Geometry: final body of the model. Coordinates: model frame, mm. Round coordinates to 2 decimals unless told otherwise and drop trailing zeros. Loops run counter-clockwise (first coordinate to the right, second up) from the corner with the lowest first, then second, coordinate; pieces in that order, holes last. Notation, with made-up numbers: (-4.5, 84) - (51.5, 84) arc R33 cw to (51.5, 112) - close; hole circle Ø6 at (20, 87.25). An arc over 180 degrees is marked (long way). Answer as CSV lines item,"result".
from build123d import *

# Parameters (mm, degrees)
BOSS_EXTRUDE1_DEPTH = 2.54


with BuildPart() as part:
    # Model → Boss-Extrude1 (new body)
    with BuildSketch(Plane.XY):
        with BuildLine():
            Line((0.837402515, 4.194701871), (0.812002515, 4.238232391))
            ThreePointArc((0.812002515, 4.238232391), (0.774103936, 4.334279035), (0.761202515, 4.436723231))
            ThreePointArc((0.761202515, 4.436723231), (0.774103936, 4.539167428), (0.812002515, 4.635214071))
            Line((0.812002515, 4.635214071), (0.837402515, 4.678744591))
            Line((0.837402515, 4.678744591), (0.862802515, 4.715127551))
            Line((0.862802515, 4.715127551), (0.888202515, 4.746935971))
            Line((0.888202515, 4.746935971), (0.913602515, 4.775495731))
            Line((0.913602515, 4.775495731), (0.939002515, 4.801589151))
            Line((0.939002515, 4.801589151), (0.964402515, 4.825726771))
            Line((0.964402515, 4.825726771), (0.989802515, 4.848266731))
            Line((0.989802515, 4.848266731), (1.015202515, 4.869465571))
            ThreePointArc((1.015202515, 4.869465571), (1.089772897, 4.925535764), (1.167602515, 4.976986311))
            Line((1.167602515, 4.976986311), (1.193002515, 4.992508251))
            ThreePointArc((1.193002515, 4.992508251), (1.305754767, 5.055617229), (1.421602515, 5.112845831))
            Line((1.421602515, 5.112845831), (1.447002515, 5.124547611))
            ThreePointArc((1.447002515, 5.124547611), (1.598149319, 5.189132356), (1.751802515, 5.247503931))
            Line((1.751802515, 5.247503931), (1.777202515, 5.256564111))
            ThreePointArc((1.777202515, 5.256564111), (1.991913899, 5.32756087), (2.209002515, 5.390917411))
            Line((2.209002515, 5.390917411), (2.234402515, 5.397856691))
            ThreePointArc((2.234402515, 5.397856691), (2.512823075, 5.468426298), (2.793202515, 5.530759651))
            Line((2.793202515, 5.530759651), (2.818602515, 5.536032691))
            ThreePointArc((2.818602515, 5.536032691), (3.18604982, 5.606262809), (3.555202515, 5.666893491))
            Line((3.555202515, 5.666893491), (3.580602515, 5.670744131))
            ThreePointArc((3.580602515, 5.670744131), (4.049820252, 5.735370933), (4.520402515, 5.789169091))
            Line((4.520402515, 5.789169091), (4.545802515, 5.791795451))
            ThreePointArc((4.545802515, 5.791795451), (5.129518216, 5.845119064), (5.714202515, 5.886491731))
            Line((5.714202515, 5.886491731), (5.739602515, 5.888043671))
            ThreePointArc((5.739602515, 5.888043671), (6.437840457, 5.923508303), (7.136602515, 5.946433191))
            Line((7.136602515, 5.946433191), (7.162002515, 5.947052951))
            ThreePointArc((7.162002515, 5.947052951), (7.987453434, 5.959786425), (8.813002515, 5.959509111))
            Line((8.813002515, 5.959509111), (8.838402515, 5.959313531))
            ThreePointArc((8.838402515, 5.959313531), (9.791045496, 5.944671622), (10.743402515, 5.917119051))
            Line((10.743402515, 5.917119051), (10.768802515, 5.916224971))
            ThreePointArc((10.768802515, 5.916224971), (11.874009843, 5.869976991), (12.978602515, 5.810840371))
            Line((12.978602515, 5.810840371), (13.004002515, 5.809341771))
            ThreePointArc((13.004002515, 5.809341771), (14.249024434, 5.729100435), (15.493202515, 5.636692891))
            Line((15.493202515, 5.636692891), (15.518602515, 5.634691371))
            ThreePointArc((15.518602515, 5.634691371), (16.763614783, 5.531321058), (18.007802486, 5.418458634))
            Line((18.007802486, 5.418458634), (18.134802481, 5.406436814))
            ThreePointArc((18.134802481, 5.406436814), (19.379819615, 5.283861478), (20.624002515, 5.153089591))
            Line((20.624002515, 5.153089591), (20.649402515, 5.150333691))
            ThreePointArc((20.649402515, 5.150333691), (21.894471689, 5.011181274), (23.138602515, 4.863875031))
            Line((23.138602515, 4.863875031), (23.164002515, 4.860781311))
            ThreePointArc((23.164002515, 4.860781311), (24.409193854, 4.704533833), (25.653202485, 4.539133495))
            Line((25.653202485, 4.539133495), (26.161202515, 4.468727231))
            ThreePointArc((26.161202515, 4.468727231), (26.191266445, 4.466787161), (26.189326375, 4.436723231))
            ThreePointArc((26.189326375, 4.436723231), (26.191266445, 4.406659301), (26.161202515, 4.404719231))
            Line((26.161202515, 4.404719231), (25.653202485, 4.334312967))
            ThreePointArc((25.653202485, 4.334312967), (24.409193854, 4.168912629), (23.164002515, 4.012665151))
            Line((23.164002515, 4.012665151), (23.138602515, 4.009571431))
            ThreePointArc((23.138602515, 4.009571431), (21.894471689, 3.862265188), (20.649402515, 3.723112771))
            Line((20.649402515, 3.723112771), (20.624002515, 3.720356871))
            ThreePointArc((20.624002515, 3.720356871), (19.379819615, 3.589584984), (18.134802481, 3.467009648))
            Line((18.134802481, 3.467009648), (18.007802486, 3.454987828))
            ThreePointArc((18.007802486, 3.454987828), (16.763614783, 3.342125404), (15.518602515, 3.238755091))
            Line((15.518602515, 3.238755091), (15.493202515, 3.236753571))
            ThreePointArc((15.493202515, 3.236753571), (14.249024434, 3.144346027), (13.004002515, 3.064104691))
            Line((13.004002515, 3.064104691), (12.978602515, 3.062606091))
            ThreePointArc((12.978602515, 3.062606091), (11.874009843, 3.003469471), (10.768802515, 2.957221491))
            Line((10.768802515, 2.957221491), (10.743402515, 2.956327411))
            ThreePointArc((10.743402515, 2.956327411), (9.791045496, 2.92877484), (8.838402515, 2.914132931))
            Line((8.838402515, 2.914132931), (8.813002515, 2.913937351))
            ThreePointArc((8.813002515, 2.913937351), (7.987453434, 2.913660037), (7.162002515, 2.926393511))
            Line((7.162002515, 2.926393511), (7.136602515, 2.927013271))
            ThreePointArc((7.136602515, 2.927013271), (6.437840457, 2.949938159), (5.739602515, 2.985402791))
            Line((5.739602515, 2.985402791), (5.714202515, 2.986954731))
            ThreePointArc((5.714202515, 2.986954731), (5.129518216, 3.028327398), (4.545802515, 3.081651011))
            Line((4.545802515, 3.081651011), (4.520402515, 3.084277371))
            ThreePointArc((4.520402515, 3.084277371), (4.049820252, 3.138075529), (3.580602515, 3.202702331))
            Line((3.580602515, 3.202702331), (3.555202515, 3.206552971))
            ThreePointArc((3.555202515, 3.206552971), (3.18604982, 3.267183653), (2.818602515, 3.337413771))
            Line((2.818602515, 3.337413771), (2.793202515, 3.342686811))
            ThreePointArc((2.793202515, 3.342686811), (2.512823075, 3.405020164), (2.234402515, 3.475589771))
            Line((2.234402515, 3.475589771), (2.209002515, 3.482529051))
            ThreePointArc((2.209002515, 3.482529051), (1.991913899, 3.545885592), (1.777202515, 3.616882351))
            Line((1.777202515, 3.616882351), (1.751802515, 3.625942531))
            ThreePointArc((1.751802515, 3.625942531), (1.598149319, 3.684314106), (1.447002515, 3.748898851))
            Line((1.447002515, 3.748898851), (1.421602515, 3.760600631))
            ThreePointArc((1.421602515, 3.760600631), (1.305754767, 3.817829233), (1.193002515, 3.880938211))
            Line((1.193002515, 3.880938211), (1.167602515, 3.896460151))
            ThreePointArc((1.167602515, 3.896460151), (1.089772897, 3.947910699), (1.015202515, 4.003980891))
            Line((1.015202515, 4.003980891), (0.989802515, 4.025179731))
            Line((0.989802515, 4.025179731), (0.964402515, 4.047719691))
            Line((0.964402515, 4.047719691), (0.939002515, 4.071857311))
            Line((0.939002515, 4.071857311), (0.913602515, 4.097950731))
            Line((0.913602515, 4.097950731), (0.888202515, 4.126510491))
            Line((0.888202515, 4.126510491), (0.862802515, 4.158318911))
            Line((0.862802515, 4.158318911), (0.837402515, 4.194701871))
        make_face()
    extrude(amount=BOSS_EXTRUDE1_DEPTH)


solid = part.part
(1) Section B-B (x = 10.5). Output: boundary loops of the cut face in (y, z).
Findings below:
outline,"(2.95, 0) - (5.93, 0) - (5.93, 2.54) - (2.95, 2.54) - close"
(2) Section A-A (x = 6). Output: boundary loops of the cut face in (y, z), and give its area (3 significant figures).
Findings below:
outline,"(2.97, 0) - (5.9, 0) - (5.9, 2.54) - (2.97, 2.54) - close"
area,"7.45 mm2"
(3) Material intervals for line 1 along Y through (x, z) = (13.25, 0.3); line 2 along Y through (x, z) = (7.75, 0.2), sorted ascending.
Findings below:
line 1,"3.08 to 5.79"
line 2,"2.92 to 5.96"
